Verification items for the finished model (mm, model axes). Round coordinates to 2 decimals unless told otherwise and drop trailing zeros. Write each loop counter-clockwise with the first axis right and the second up, starting at its lowest first coordinate (ties: lowest second). Pieces come first, ordered by that corner, then holes. Notation, with made-up numbers: (-37, 57.5) - (1, 57.5) arc R37 cw to (1, 96.5) - close; hole circle Ø11 at (38, -6.5). An arc over 180 degrees is marked (long way). Answer as a JSON object with one key per item and string values. Group by question number.
1) Section check B-B (x = 44.45). Enter the section's corners in (y, z), then the cut area to 3 significant figures.
2) Thickness scan on line 1 (X direction, y = 1.5, z = -19.05); line 2 (X direction, y = 3, z = -40); line 3 (Z direction, x = -1.5, y = -4). Record the ranges inside material, lowest first.
3) Section check C-C (y = -2.5). Enter the section's corners in (x, z).
4) Mould release check, pull along Z, two halves, no side actions. Record for faces 1 (the cylindrical face through (-61.69, -0.09, -48.89)), 2 (the cylindrical face through (-61.69, 0.09, 48.89)), 3 (the cylindrical face through (-38.154, -0.089, -19.877)): +Z half, -Z half, draft (parallel to the pull), parting line (faces both ways), or undercut.
5) Section check D-D (x = -41). Enter the section's corners in (y, z), then the cut area to 3 significant figures.
6) Section check A-A (x = 0). Enter the section's corners in (y, z).
```python
from build123d import *

# Parameters (mm, degrees)
SKETCH1_W           = 127
SKETCH1_H           = 101.6
SKETCH1_R           = 3.2639
SKETCH1_R_2         = 6.35
BOSS_EXTRUDE1_DEPTH = 6.35
FILLET1_R           = 6.35


with BuildPart() as part:
    # Sketch1 → Boss-Extrude1 (new, symmetric)
    with BuildSketch(Plane(origin=(0, 0, 0), x_dir=(1, 0, 0), z_dir=(0, 1, 0))):
        Rectangle(SKETCH1_W, SKETCH1_H)
        with Locations(Location((0, 23.368, 0), (0, 0, 270))):
            Circle(SKETCH1_R, mode=Mode.SUBTRACT)
        with Locations(Location((0, 40.386, 0), (0, 0, 270))):
            Circle(SKETCH1_R, mode=Mode.SUBTRACT)
        with Locations(Location((0, -23.368, 0), (0, 0, 90))):
            Circle(SKETCH1_R, mode=Mode.SUBTRACT)
        with Locations(Location((0, -40.386, 0), (0, 0, 90))):
            Circle(SKETCH1_R, mode=Mode.SUBTRACT)
        with Locations(Location((-44.45, 19.05, 0), (0, 0, 270))):
            Circle(SKETCH1_R_2, mode=Mode.SUBTRACT)
        with Locations(Location((44.45, 19.05, 0), (0, 0, 270))):
            Circle(SKETCH1_R_2, mode=Mode.SUBTRACT)
    extrude(amount=BOSS_EXTRUDE1_DEPTH, both=True)

    # Fillet1
    fillet1_edges = [part.edges().sort_by_distance(p)[0] for p in [
        (63.5, 0, 50.8),
        (-63.5, 0, 50.8),
        (-63.5, 0, -50.8),
        (63.5, 0, -50.8),
    ]]
    fillet(fillet1_edges, radius=FILLET1_R)


solid = part.part
```
Returned:
{
 "1": {"outline": "(-6.35, -50.8) - (6.35, -50.8) - (6.35, -25.4) - (-6.35, -25.4) - close; (-6.35, -12.7) - (6.35, -12.7) - (6.35, 50.8) - (-6.35, 50.8) - close", "area": "1,130 mm2"},
 "2": {"line 1": "-63.5 to -50.8, -38.1 to 38.1, 50.8 to 63.5", "line 2": "-63.5 to -3.24, 3.24 to 63.5", "line 3": "-50.8 to -43.28, -37.49 to -26.27, -20.47 to 20.47, 26.27 to 37.49, 43.28 to 50.8"},
 "3": {"outline": "(-63.5, -44.45) arc R6.35 ccw to (-57.15, -50.8) - (57.15, -50.8) arc R6.35 ccw to (63.5, -44.45) - (63.5, 44.45) arc R6.35 ccw to (57.15, 50.8) - (-57.15, 50.8) arc R6.35 ccw to (-63.5, 44.45) - close; hole circle Ø12.7 at (-44.45, -19.05); hole circle Ø6.53 at (0, -40.39); hole circle Ø6.53 at (0, -23.37); hole circle Ø6.53 at (0, 23.37); hole circle Ø6.53 at (0, 40.39); hole circle Ø12.7 at (44.45, -19.05)"},
 "4": {"face 1": "-Z half", "face 2": "+Z half", "face 3": "undercut"},
 "5": {"outline": "(-6.35, -50.8) - (6.35, -50.8) - (6.35, -24.38) - (-6.35, -24.38) - close; (-6.35, -13.72) - (6.35, -13.72) - (6.35, 50.8) - (-6.35, 50.8) - close", "area": "1,150 mm2"},
 "6": {"outline": "(-6.35, -50.8) - (6.35, -50.8) - (6.35, -43.65) - (-6.35, -43.65) - close; (-6.35, -37.12) - (6.35, -37.12) - (6.35, -26.63) - (-6.35, -26.63) - close; (-6.35, -20.1) - (6.35, -20.1) - (6.35, 20.1) - (-6.35, 20.1) - close; (-6.35, 26.63) - (6.35, 26.63) - (6.35, 37.12) - (-6.35, 37.12) - close; (-6.35, 43.65) - (6.35, 43.65) - (6.35, 50.8) - (-6.35, 50.8) - close"}
}
